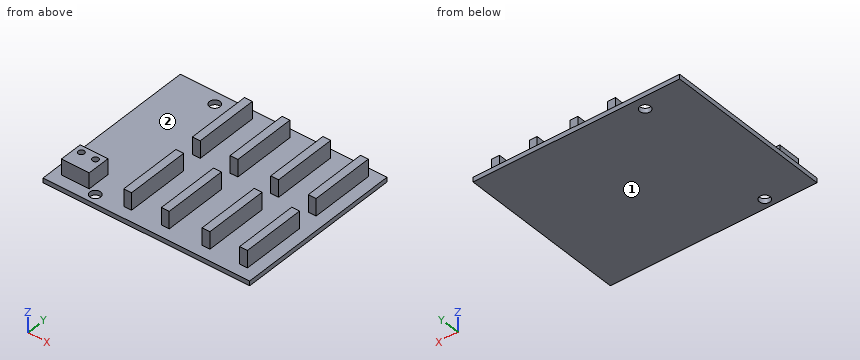
```python
from build123d import *

# Parameters (mm, degrees)
SKETCH075_W                     = 66
SKETCH075_H                     = 54
PAD041_DEPTH                    = 1.5
SKETCH076_W                     = 2.5
SKETCH076_H                     = 20.5
PAD042_DEPTH                    = 7
SKETCH076_LINEARPATTERN002_2_W  = 2.5
SKETCH076_LINEARPATTERN002_2_H  = 20.5
PAD042_LINEARPATTERN002_2_DEPTH = 7
LINEARPATTERN003_COUNT          = 2
LINEARPATTERN003_PITCH          = 27
SKETCH077_W                     = 8.886057
SKETCH077_H                     = 7.374495
SKETCH077_R                     = 0.972187
PAD043_DEPTH                    = 5
SKETCH078_R                     = 1.7
HOLE_DEPTH                      = 25


with BuildPart() as part:
    # Sketch075 → Pad041 (new body)
    with BuildSketch(Plane.XY):
        Rectangle(SKETCH075_W, SKETCH075_H)
    extrude(amount=PAD041_DEPTH)

    # Sketch076 → Pad042 (join)
    with BuildSketch(Plane(origin=(-3, -13, 0), x_dir=(1, 0, 0), z_dir=(0, 0, 1))):
        with Locations((-6, 0)):
            Rectangle(SKETCH076_W, SKETCH076_H)
        with Locations((6, 0)):
            Rectangle(SKETCH076_W, SKETCH076_H)
    pad042 = extrude(amount=PAD042_DEPTH)

    # Sketch076 LinearPattern002 2 → Pad042 LinearPattern002 2 (add)
    with BuildSketch(Plane(origin=(22, -13, 0), x_dir=(1, 0, 0), z_dir=(0, 0, 1))):
        with Locations((-6, 0)):
            Rectangle(SKETCH076_LINEARPATTERN002_2_W, SKETCH076_LINEARPATTERN002_2_H)
        with Locations((6, 0)):
            Rectangle(SKETCH076_LINEARPATTERN002_2_W, SKETCH076_LINEARPATTERN002_2_H)
    pad042_linearpattern002_2 = extrude(amount=PAD042_LINEARPATTERN002_2_DEPTH)

    # LinearPattern003: Pad042, Pad042 LinearPattern002 2 ×2
    with Locations(*[(0, i * LINEARPATTERN003_PITCH, 0) for i in range(1, LINEARPATTERN003_COUNT)]):
        add(pad042)
        add(pad042_linearpattern002_2)

    # Sketch077 → Pad043 (join)
    with BuildSketch(Plane.XY.offset(1.5)):
        with Locations((-25.795806, -19.485859)):
            Rectangle(SKETCH077_W, SKETCH077_H)
        with Locations((-28.09366, -17.955694)):
            Circle(SKETCH077_R, mode=Mode.SUBTRACT)
        with Locations((-23.577271, -17.955694)):
            Circle(SKETCH077_R, mode=Mode.SUBTRACT)
    extrude(amount=PAD043_DEPTH)

    # Sketch078 → Hole (cut)
    with BuildSketch(Plane.XY.offset(1.5)):
        with Locations((-18.75, 23)):
            Circle(SKETCH078_R)
        with Locations((-18.75, -24)):
            Circle(SKETCH078_R)
    extrude(amount=-HOLE_DEPTH, mode=Mode.SUBTRACT)


solid = part.part
```
Check sheet for the modelled part. Datum: model origin and axes. Units: mm. Face numbers are marked on the shaded views. Give positions to 0.01 mm unless a question says otherwise; leave off trailing zeros. Order: outer loops, then holes, each group sorted by start corner. A loop starts at its lowest first (then second) coordinate and runs counter-clockwise, first axis right, second up. Notation, with made-up numbers: (-28.75, -23.5) -> (20.25, -23.5) arc R25 ccw to (20.25, -10.5) -> close; hole circle Ø8 at (-29.75, 53). An arc over 180 degrees is marked (long way). Use CSV: the item, a comma, the result in double quotes. Start each with the question number.
1) Sectioned sample at A-A, the plane x = -18.75. Record the boundary of the cut face in (y, z), plus the area to 3 significant figures.
2) Sectioned sample at D-D, the plane x = 16. Record the boundary of the cut face in (y, z).
3) Sectioned sample at C-C, the plane y = 8.5. Record the boundary of the cut face in (x, z), plus the area to 3 significant figures.
4) Go/stop test with flat-tipped pins: P1, Ø1.5, axis at x = -16.5, y = -21.5, coming from the +Z side; P2, Ø1.2, axis at x = 3, z = 3, coming from the -Y side; P3, Ø1.5, axis at x = -28, z = 3, coming from the +Y side; P4, Ø2, axis at x = -18.75, y = -24, coming from the -Z side. Record where each tip stops, or that it passes through.
5) Material ranges on line 1 (X direction, y = -19, z = 2.25); line 2 (X direction, y = 6, z = 2.25); line 3 (Y direction, x = -18.75, z = 0.6), recorded low to high. Write a range as from..to.
6) Mould release check, pull along X, two halves, no side actions. Record for the marked faces 1 and 2: released by +X, released by -X, zero draft, split by the parting line, or undercut.
7) Sectioned sample at B-B, the plane y = -24. Record the boundary of the cut face in (x, z), plus the area to 3 significant figures.
Recorded:
1,outline,"(-27, 0) -> (-25.7, 0) -> (-25.7, 1.5) -> (-27, 1.5) -> close; (-22.3, 0) -> (21.3, 0) -> (21.3, 1.5) -> (-22.3, 1.5) -> close; (24.7, 0) -> (27, 0) -> (27, 1.5) -> (24.7, 1.5) -> close"
1,area,"70.8 mm2"
2,outline,"(-27, 0) -> (27, 0) -> (27, 1.5) -> (24.25, 1.5) -> (24.25, 7) -> (3.75, 7) -> (3.75, 1.5) -> (-2.75, 1.5) -> (-2.75, 7) -> (-23.25, 7) -> (-23.25, 1.5) -> (-27, 1.5) -> close"
3,outline,"(-33, 0) -> (33, 0) -> (33, 1.5) -> (29.25, 1.5) -> (29.25, 7) -> (26.75, 7) -> (26.75, 1.5) -> (17.25, 1.5) -> (17.25, 7) -> (14.75, 7) -> (14.75, 1.5) -> (4.25, 1.5) -> (4.25, 7) -> (1.75, 7) -> (1.75, 1.5) -> (-7.75, 1.5) -> (-7.75, 7) -> (-10.25, 7) -> (-10.25, 1.5) -> (-33, 1.5) -> close"
3,area,"154 mm2"
4,P1,"z = 1.5"
4,P2,"y = -23.25"
4,P3,"y = -15.8"
4,P4,"through"
5,line 1,"-30.24..-21.35, -10.25..-7.75, 1.75..4.25, 14.75..17.25, 26.75..29.25"
5,line 2,"-10.25..-7.75, 1.75..4.25, 14.75..17.25, 26.75..29.25"
5,line 3,"-27..-25.7, -22.3..21.3, 24.7..27"
6,face 1,"zero draft"
6,face 2,"undercut"
7,outline,"(-33, 0) -> (-20.45, 0) -> (-20.45, 1.5) -> (-33, 1.5) -> close; (-17.05, 0) -> (33, 0) -> (33, 1.5) -> (-17.05, 1.5) -> close"
7,area,"93.9 mm2"
